The listing builds one solid part. Answer for the finished solid, in the listing's coordinates (mm). A direction names the side the tool comes from. Round coordinates to 2 decimals unless told otherwise and drop trailing zeros. Loops run counter-clockwise (first coordinate to the right, second up) from the corner with the lowest first, then second, coordinate; pieces in that order, holes last. Notation, with made-up numbers: (43, 14.5) - (95, 14.5) arc R18 cw to (95, 20.5) - close; hole circle Ø9 at (55.5, 43.25). An arc over 180 degrees is marked (long way). Write item = value, one per line. Start each with the question number.
1) Given pin 1 Ø1.3 at (x, z) = (0, 2.15) entering from -Y; pin 2 Ø1 at (y, z) = (0, -2) entering from -X; pin 3 Ø0.5 at (x, z) = (-1.5, -4.5) entering from -Y, each flat-ended and moving along its own axis, determine where each tip first touches the part or whether it passes through.
2) Section B-B, the plane x = -1.7 is taken. Determine the outline of the cut face in (y, z).
3) Section A-A, the plane z = -7.25 is taken. Determine the outline of the cut face in (x, y).
4) A tool of negligible diameter and unlimited length cuts with its end or side. For faces 1 (the flat face through (1.734, 0.162, -1.826)), 2 (the flat face through (2.081, 0.493, 2.12)), 3 (the flat face through (2.57, 0, -4.97)), 4 (the flat face through (0, -1.9, 2)), 5 (the flat face through (2.513, 0.32, -4.606)), from which of +Z, -Z, +X, -X, +Y, -Y can it reach the whole face along a straight path? Write none if from no direction.
5) Straight lines are drawn through the part: line 1 along Z through (x, y) = (0, -2.1); line 2 along Y through (x, z) = (-1, 3.25). For each, find the intervals that lie inside material, in ascending order.
6) Section C-C, the plane z = 2.15 is taken. Determine the outline of the cut face in (x, y), and give its area (3 significant figures).
7) For a pull along Z with two mould halves and no side action, classify faces 6 (the flat face through (0.03, -0.84, 4.24)), 7 (the flat face through (2.09, 0.16, -1.69)), 8 (the flat face through (-2.57, 0, -4.97)) as released by +Z, released by -Z, zero draft, split by the parting line, or undercut.
8) Section D-D, the plane y = -0.75 is taken. Determine the outline of the cut face in (x, z).
from build123d import *

# Parameters (mm, degrees)
BOSS_EXTRUDE1_DEPTH = 4.3
SKETCH2_W           = 0.36
SKETCH2_H           = 0.32
SKETCH2_4_W         = 0.36
SKETCH2_4_H         = 0.32
BOSS_EXTRUDE2_DEPTH = 10
FILLET1_R           = 0.1
SKETCH4_R           = 0.8
CUT_EXTRUDE1_DEPTH  = 0.25
CUT_EXTRUDE2_DEPTH  = 5
CUT_EXTRUDE3_DEPTH  = 5
CUT_EXTRUDE4_DEPTH  = 5
CUT_EXTRUDE6_DEPTH  = 5
SKETCH4_3_R         = 0.8
CUT_EXTRUDE8_DEPTH  = 0.3


with BuildPart() as part:
    # Sketch1 → Boss-Extrude1 (new body)
    with BuildSketch(Plane.XY):
        with BuildLine():
            Line((-1.959591794, 1), (-2.2, 0))
            ThreePointArc((-2.2, 0), (0, -2.2), (2.2, 0))
            Line((2.2, 0), (1.959591794, 1))
            Line((1.959591794, 1), (-1.959591794, 1))
        make_face()
    extrude(amount=BOSS_EXTRUDE1_DEPTH)

    # Sweep1: sweep along a curve in space
    with BuildLine() as sweep1_path:
        Line((1.27, 0.16, 0), (1.27, 0.16, -1))
        Line((1.27, 0.16, -1), (2.54, 0.16, -2.5))
        Line((2.54, 0.16, -10), (2.54, 0.16, -2.5))
    # Sketch2 → Sweep1 (sweep)
    with BuildSketch(Plane.XY):
        with Locations((1.27, 0.16)):
            Rectangle(SKETCH2_W, SKETCH2_H)
    sweep1 = sweep(path=sweep1_path.line, transition=Transition.RIGHT)

    # Mirror1: Sweep1 across plane
    add(sweep1.mirror(Plane(origin=(0, 0, 0), x_dir=(0, 0, 1), z_dir=(1, 0, 0))))

    # Sketch2_4 → Boss-Extrude2 (add)
    with BuildSketch(Plane.XY):
        with Locations((0, 0.16)):
            Rectangle(SKETCH2_4_W, SKETCH2_4_H)
    extrude(amount=-BOSS_EXTRUDE2_DEPTH)

    # Fillet1
    fillet1_edges = [part.edges().sort_by_distance(p)[0] for p in [
        (2.36, 0.16, -10),
        (2.54, 0, -10),
        (2.72, 0.16, -10),
        (2.54, 0.32, -10),
        (-2.72, 0.16, -10),
        (-2.54, 0, -10),
        (-2.36, 0.16, -10),
        (-2.54, 0.32, -10),
        (0, 0, -10),
        (-0.18, 0.16, -10),
        (0.18, 0.16, -10),
        (0, 0.32, -10),
    ]]
    fillet(fillet1_edges, radius=FILLET1_R)

    # Sketch4 → Cut-Extrude1 (cut)
    with BuildSketch(Plane(origin=(0, -2.2, 0), x_dir=(1, 0, 0), z_dir=(0, 1, 0))):
        with Locations((0, -2.15)):
            Circle(SKETCH4_R)
    extrude(amount=CUT_EXTRUDE1_DEPTH, mode=Mode.SUBTRACT)

    # Sketch5 → Cut-Extrude2 (cut)
    with BuildSketch(Plane(origin=(2.2, 0, 0), x_dir=(0, 0, -1), z_dir=(1, 0, 0))):
        Polygon((-4.3, 1), (-4.14, 1), (-4.3, 0), align=None)
    extrude(amount=-CUT_EXTRUDE2_DEPTH, mode=Mode.SUBTRACT)

    # Sketch6 → Cut-Extrude3 (cut)
    with BuildSketch(Plane(origin=(2.2, 0, 0), x_dir=(0, 0, -1), z_dir=(1, 0, 0))):
        Polygon((-4.3, 0), (-4.14, -2.2), (-4.3, -2.2), align=None)
    extrude(amount=-CUT_EXTRUDE3_DEPTH, mode=Mode.SUBTRACT)

    # Sketch7 → Cut-Extrude4 (cut)
    with BuildSketch(Plane(origin=(2.2, 0, 0), x_dir=(0, 0, -1), z_dir=(1, 0, 0))):
        Polygon((0, 0), (0, -2.2), (-0.16, -2.2), align=None)
    extrude(amount=-CUT_EXTRUDE4_DEPTH, mode=Mode.SUBTRACT)

    # Sketch8 → Cut-Extrude6 (cut)
    with BuildSketch(Plane(origin=(2.2, 0, 0), x_dir=(0, 0, -1), z_dir=(1, 0, 0))):
        Polygon((0, 0.32), (0, 1), (-0.16, 1), align=None)
    extrude(amount=-CUT_EXTRUDE6_DEPTH, mode=Mode.SUBTRACT)

    # Sketch4_3 → Cut-Extrude8 (cut)
    with BuildSketch(Plane(origin=(0, -2.2, 0), x_dir=(1, 0, 0), z_dir=(0, 1, 0))):
        with Locations((0, -2.15)):
            Circle(SKETCH4_3_R)
    extrude(amount=CUT_EXTRUDE8_DEPTH, mode=Mode.SUBTRACT)


solid = part.part
Geometry check:
q1.pin_1 = -1.9
q1.pin_2 = -2.72
q1.pin_3 = through
q2.outline = (-1.4, 0.1) - (0, 0) - (0.32, 0) - (1, 0.16) - (1, 4.14) - (0, 4.3) - (-1.4, 4.2) - close; (0, -1.79) - (0.32, -1.79) - (0.32, -1.23) - (0, -1.23) - close
q3.outline = (-2.72, 0) - (-2.36, 0) - (-2.36, 0.32) - (-2.72, 0.32) - close; (-0.18, 0) - (0.18, 0) - (0.18, 0.32) - (-0.18, 0.32) - close; (2.36, 0) - (2.72, 0) - (2.72, 0.32) - (2.36, 0.32) - close
q4.face_1 = -Z, +Y, -Y
q4.face_2 = +Z, +X, +Y
q4.face_3 = -Z, +X, -X, -Y
q4.face_4 = -Y
q4.face_5 = -Z, +X, -X, +Y
q5.line_1 = 0.15 to 1.35, 2.95 to 4.15
q5.line_2 = -1.96 to 1
q6.outline = (-2.2, 0) arc R2.2 ccw to (-0.8, -2.05) - (-0.8, -1.9) - (0.8, -1.9) - (0.8, -2.05) arc R2.2 ccw to (2.2, 0) - (1.96, 1) - (-1.96, 1) - close
q6.area = 11.4 mm2
q7.face_6 = released by +Z
q7.face_7 = undercut
q7.face_8 = zero draft
q8.outline = (-2.07, 0.05) - (2.07, 0.05) - (2.07, 4.25) - (-2.07, 4.25) - close
